```python
from build123d import *

# Parameters (mm, degrees)
F0_R     = 2.9315059489
F0_R_2   = 4.9577082706
F0_R_3   = 3.0008121714
F1_DEPTH = 6.35


with BuildPart() as f1:
    # F0 (on Top) → F1 (new body)
    with BuildSketch(Plane.XY):
        with BuildLine():
            ThreePointArc((-31.111174148, 10.771264197), (-5.4612938069, -32.4668994396), (32.9230206583, 0))
            ThreePointArc((32.9230206583, 0), (31.6741105539, 8.9819825144), (28.0221331774, 17.282515484))
            ThreePointArc((28.0221331774, 17.282515484), (11.0885388977, 15.9908350993), (6.3616782796, 32.3025438431))
            ThreePointArc((6.3616782796, 32.3025438431), (-4.6856163495, 32.5878856125), (-15.2049900361, 29.2016021353))
            ThreePointArc((-15.2049900361, 29.2016021353), (-13.2179182524, 25.5820794163), (-12.5301148045, 21.510676046))
            ThreePointArc((-12.5301148045, 21.510676046), (-18.7221234211, 10.7799871913), (-31.111174148, 10.771264197))
        make_face()
        with BuildLine():
            ThreePointArc((17.930932343, -15.3499655426), (0.2098643008, -26.5919373772), (-16.5725294501, -13.9915626496))
            Line((-16.5725294501, -13.9915626496), (-11.4105949178, -9.6446694806))
            ThreePointArc((-11.4105949178, -9.6446694806), (0.750091805, -15.8180913269), (12.7689968795, -9.3729877844))
            Line((12.7689968795, -9.3729877844), (17.930932343, -15.3499655426))
        make_face(mode=Mode.SUBTRACT)
        with Locations((-14.3990833312, 8.286264725)):
            Circle(F0_R, mode=Mode.SUBTRACT)
        with Locations((0, 5.0260950811)):
            Circle(F0_R_2, mode=Mode.SUBTRACT)
        with Locations((13.0406813696, 7.4712228961)):
            Circle(F0_R_3, mode=Mode.SUBTRACT)
        with BuildLine():
            ThreePointArc((6.3616782796, 32.3025438431), (11.0885388977, 15.9908350993), (28.0221331774, 17.282515484))
            ThreePointArc((28.0221331774, 17.282515484), (18.760648591, 27.0548212656), (6.3616782796, 32.3025438431))
        make_face()
        with BuildLine():
            ThreePointArc((6.3616782796, 32.3025438431), (18.760648591, 27.0548212656), (28.0221331774, 17.282515484))
            ThreePointArc((28.0221331774, 17.282515484), (31.1293093852, 21.7360538154), (32.2244168983, 27.0548212656))
            ThreePointArc((32.2244168983, 27.0548212656), (21.4379787454, 40.2497051331), (6.3616782796, 32.3025438431))
        make_face()
        with BuildLine():
            ThreePointArc((-15.2049900361, 29.2016021353), (-34.3070925434, 29.6085146222), (-31.111174148, 10.771264197))
            ThreePointArc((-31.111174148, 10.771264197), (-24.9242072153, 21.510676046), (-15.2049900361, 29.2016021353))
        make_face()
        with BuildLine():
            ThreePointArc((-15.2049900361, 29.2016021353), (-24.9242072153, 21.510676046), (-31.111174148, 10.771264197))
            ThreePointArc((-31.111174148, 10.771264197), (-18.7221234211, 10.7799871913), (-12.5301148045, 21.510676046))
            ThreePointArc((-12.5301148045, 21.510676046), (-13.2179182524, 25.5820794163), (-15.2049900361, 29.2016021353))
        make_face()
    extrude(amount=F1_DEPTH)


solid = f1.part
```
The listing builds one solid part. Answer for the finished solid, in the listing's coordinates (mm). A direction names the side the tool comes from. Give positions to 0.01 mm unless a question says otherwise; leave off trailing zeros. Loops run counter-clockwise (first coordinate to the right, second up) from the corner with the lowest first, then second, coordinate; pieces in that order, holes last. Notation, with made-up numbers: (19.5, -17) - (32.5, -17) arc R19 cw to (32.5, 0) - close; hole circle Ø8 at (21.25, 75.5). An arc over 180 degrees is marked (long way). Answer as CSV lines item,"result". Start each with the question number.
Item 1: A cutting plane is placed at A-A on x = 0. Determine the outline of the cut face in (y, z), then the cut area to 3 significant figures.
Item 2: This flat-tipped pin is pushed along its axis until it touches: pin 1 (3 mm diameter, centred on x = -28, z = 3, fed in from -Y). Where does it stop, or does it pass through?
Item 3: For faces 3 (the face through (15.314, -12.32, 3.131)), 4 (the face through (-4.53, 32.61, 3.13)), determine the directions among +Z, -Z, +X, -X, +Y, -Y from which every point of the face is accessible in a straight line to the end or side of a thin tool.
Item 4: The mould has two halves that part along X. Classify faces 1 (the face through (5.1, 4.3, 6.35)), 2 (the face through (-14.03, -11.85, 3.13)): +X half, -X half, draft (parallel to the pull), parting line (faces both ways), or undercut.
Item 5: A cutting plane is placed at D-D on y = 35.5. Determine the outline of the cut face in (x, z), then the cut area to 3 significant figures.
Item 6: Find the intervals of material crossed by line 1 (X direction, y = -10.5, z = 1.5); line 2 (X direction, y = -14, z = 0.5); line 3 (Y direction, x = -14, z = 1.5), in increasing order. Write a range as from..to.
Item 7: A cutting plane is placed at C-C on z = 4.5. Determine the outline of the cut face in (x, y) (1 decimal).
Item 8: A cutting plane is placed at B-B on x = 8.5. Determine the outline of the cut face in (y, z), then the cut area to 3 significant figures.
Found:
1,outline,"(-32.92, 0) - (-26.58, 0) - (-26.58, 6.35) - (-32.92, 6.35) - close; (-15.81, 0) - (0.07, 0) - (0.07, 6.35) - (-15.81, 6.35) - close; (9.98, 0) - (32.92, 0) - (32.92, 6.35) - (9.98, 6.35) - close"
1,area,"287 mm^2"
2,pin 1,"stops at y = -19.54"
3,face 3,"+Z, -Z"
3,face 4,"+Z, -Z, +Y"
4,face 1,"draft"
4,face 2,"undercut"
5,outline,"(8.27, 0) - (29.25, 0) - (29.25, 6.35) - (8.27, 6.35) - close"
5,area,"133 mm^2"
6,line 1,"x = -31.2..-12.43, -10.75..11.92, 13.74..31.2"
6,line 2,"x = -29.8..-16.57, -6.51..7.68, 16.77..29.8"
6,line 3,"y = -29.8..-18.99, -11.83..5.38, 11.19..29.8"
7,outline,"(-31.1, 10.8) arc R32.9 ccw (long way) to (28, 17.3) arc R13.5 ccw (long way) to (6.4, 32.3) arc R32.9 ccw to (-15.2, 29.2) arc R12.4 ccw (long way) to start; hole circle Ø5.9 at (-14.4, 8.3); hole (-16.6, -14) arc R18.5 ccw to (17.9, -15.3) - (12.8, -9.4) arc R14.7 cw to (-11.4, -9.6) - close; hole circle Ø9.9 at (0, 5); hole circle Ø6 at (13, 7.5)"
8,outline,"(-31.81, 0) - (-24.99, 0) - (-24.99, 6.35) - (-31.81, 6.35) - close; (-13.51, 0) - (35.77, 0) - (35.77, 6.35) - (-13.51, 6.35) - close"
8,area,"356 mm^2"
